Build history of the part. All positions in model axes, mm. A direction names the side the tool comes from. Round coordinates to 2 decimals unless told otherwise and drop trailing zeros. Write each loop counter-clockwise with the first axis right and the second up, starting at its lowest first coordinate (ties: lowest second). Pieces come first, ordered by that corner, then holes.
1) Wall check: probe 1 along Z at (x, y) = (-28.05, -21); probe 2 along X at (y, z) = (8, 6.25); probe 3 along Y at (x, z) = (-8, 1). Give the ranges that are in metal, low to high.
2) Pull direction X, two halves, no side cores. Call faces 1 (the cylindrical face through (0, -7, 4)), 2 (the flat face through (30, -16, 4)), 3 (the flat face through (-32.5, 0, 4)): +X half, -X half, draft (parallel to the pull), parting line (faces both ways), or undercut.
3) Saw through at C-C (z = 4). State how many separate pieces and enclosed holes the cut face has, plus the area to 3 significant figures.
4) Saw through at D-D (y = -21). Write the cut outline in (x, z).
5) Flat gauge pins, fed straight in: pin 1 (4 mm diameter, centred on y = 20, z = 4.5, fed in from +X); pin 2 (2.5 mm diameter, centred on y = 13.5, z = 3, fed in from -X); pin 3 (0.8 mm diameter, centred on x = 31, z = 6, fed in from +Y); pin 4 (3.5 mm diameter, centred on x = -7.83, y = 4.56, fed in from +Z). Where does each tip first touch, or does it go through?
6) Which spindle directions (+Z, -Z, +X, -X, +Y, -Y) get a long thin tool onto all of the face, cutting with end or side? Do faces 4 (the flat face through (-27, -21, 4)), 5 (the flat face through (30, 16, 4)), 6 (the flat face through (-31, 7.5, 4)), 7 (the flat face through (31, -7.5, 4)). Say none if no direction does.
7) Saw through at B-B (y = -9). Write the cut outline in (x, z).
8) Saw through at A-A (x = 0). Write the cut outline in (y, z).
from build123d import *

# Parameters (mm, degrees)
SKETCH_1_W               = 60
SKETCH_1_H               = 48
EXTRUDE_1_DEPTH          = 8
SKETCH_2_W               = 65
SKETCH_2_H               = 15
EXTRUDE_2_DEPTH          = 8
SKETCH_3_R               = 2
CUT_EXTRUDE_1_DEPTH      = 8
PATTERN_CIRCULAR_1_COUNT = 3
SKETCH_4_R               = 1.8
CUT_EXTRUDE_2_DEPTH      = 3
MIRROR_2_COPY_1_SKETCH_R = 1.8
MIRROR_2_COPY_1_DEPTH    = 3


with BuildPart() as part:
    # 草图1 → 凸台-拉伸1 (new body)
    with BuildSketch(Plane.XY):
        Rectangle(SKETCH_1_W, SKETCH_1_H)
    extrude(amount=EXTRUDE_1_DEPTH)

    # 草图2 → 凸台-拉伸2 (add)
    with BuildSketch(Plane.XY.offset(8)):
        Rectangle(SKETCH_2_W, SKETCH_2_H)
    extrude(amount=-EXTRUDE_2_DEPTH)

    # 草图3 → 切除-拉伸1 (cut)
    with BuildSketch(Plane.XY.offset(8)):
        with Locations((0, -9)):
            Circle(SKETCH_3_R)
    cut_extrude_1 = extrude(amount=-CUT_EXTRUDE_1_DEPTH, mode=Mode.SUBTRACT)

    # 阵列(圆周)1: 切除-拉伸1 ×3 about axis
    pattern_circular_1_axis = Axis((0, 0.038436665, 0), (0, 0, 1))
    for i in range(1, PATTERN_CIRCULAR_1_COUNT):
        add(cut_extrude_1.rotate(pattern_circular_1_axis, i * 360 / PATTERN_CIRCULAR_1_COUNT), mode=Mode.SUBTRACT)

    # 草图4 → 切除-拉伸2 (cut)
    with BuildSketch(Plane(origin=(30, 0, 0), x_dir=(0, 0, -1), z_dir=(1, 0, 0))):
        with Locations(Location((-4, 21, 0), (0, 0, 90))):
            Circle(SKETCH_4_R)
    cut_extrude_2 = extrude(amount=-CUT_EXTRUDE_2_DEPTH, mode=Mode.SUBTRACT)

    # 镜向1: 切除-拉伸2 across plane
    add(cut_extrude_2.mirror(Plane.ZX), mode=Mode.SUBTRACT)

    # 镜向2: 切除-拉伸2 across plane
    add(cut_extrude_2.mirror(Plane(origin=(0, 0, 0), x_dir=(0, 0, 1), z_dir=(1, 0, 0))), mode=Mode.SUBTRACT)

    # 镜向2 copy 1 sketch → 镜向2 copy 1 (cut)
    with BuildSketch(Plane(origin=(-30, 0, 0), x_dir=(0, 0, -1), z_dir=(-1, 0, 0))):
        with Locations(Location((-4, 21, 0), (0, 0, 90))):
            Circle(MIRROR_2_COPY_1_SKETCH_R)
    extrude(amount=-MIRROR_2_COPY_1_DEPTH, mode=Mode.SUBTRACT)


solid = part.part
Evaluation:
1. probe 1: z = 0 to 2.2, 5.8 to 8
1. probe 2: x = -30 to 30
1. probe 3: y = -24 to 2.57, 6.55 to 24
2. face 1: undercut
2. face 2: +X half
2. face 3: -X half
3. separate pieces: 1
3. enclosed holes: 3
3. area: 2,870 mm2
4. outline: (-30, 0) - (30, 0) - (30, 2.2) - (27, 2.2) - (27, 5.8) - (30, 5.8) - (30, 8) - (-30, 8) - (-30, 5.8) - (-27, 5.8) - (-27, 2.2) - (-30, 2.2) - close
5. pin 1: stops at x = 30
5. pin 2: stops at x = -30
5. pin 3: stops at y = 7.5
5. pin 4: passes through
6. face 4: -X
6. face 5: +Z, -Z, +X, +Y
6. face 6: +Z, -Z, -X, +Y
6. face 7: +Z, -Z, +X, -Y
7. outline: (-30, 0) - (-2, 0) - (-2, 8) - (-30, 8) - close; (2, 0) - (30, 0) - (30, 8) - (2, 8) - close
8. outline: (-24, 0) - (-11, 0) - (-11, 8) - (-24, 8) - close; (-7, 0) - (24, 0) - (24, 8) - (-7, 8) - close
